Check sheet for the modelled part. Datum: model origin and axes. Units: mm. Face numbers are marked on the shaded views. A direction names the side the tool comes from. Give positions to 0.01 mm unless a question says otherwise; leave off trailing zeros. Order: outer loops, then holes, each group sorted by start corner. A loop starts at its lowest first (then second) coordinate and runs counter-clockwise, first axis right, second up. Notation, with made-up numbers: (3.25, 39) - (14.25, 39) arc R33 ccw to (14.25, 69) - close; hole circle Ø6 at (86, 34.5). An arc over 180 degrees is marked (long way). Answer in a Markdown table with one row per item.
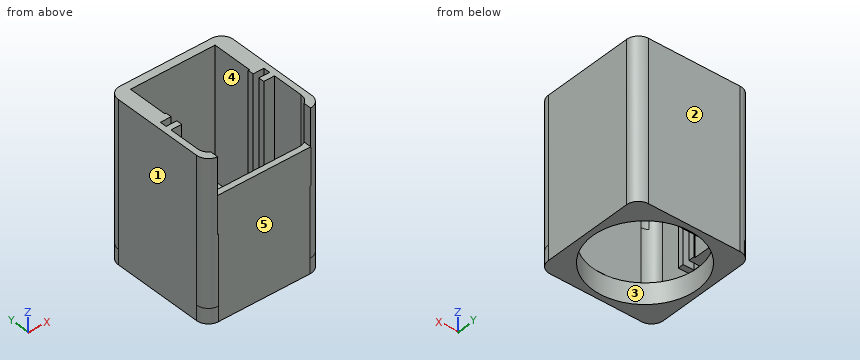
from build123d import *

# Parameters (mm, degrees)
SKETCH1_W            = 100
SKETCH1_H            = 100
BOSS_EXTRUDE1_DEPTH  = 250
SKETCH2_W            = 90
SKETCH2_H            = 90
CUT_EXTRUDE1_DEPTH   = 288.228132327
FILLET1_R            = 10.16
SKETCH3_W            = 9.3412
SKETCH3_H            = 5
BOSS_EXTRUDE2_DEPTH  = 250
SKETCH4_W            = 100
SKETCH4_H            = 125
CUT_EXTRUDE2_DEPTH   = 288.228132327
SKETCH6_W            = 90
SKETCH6_H            = 5.08
BOSS_EXTRUDE3_DEPTH  = 95
SKETCH7_R            = 45.3
CUT_EXTRUDE4_DEPTH   = 5.08
SKETCH10_R           = 48.300000047
BOSS_EXTRUDE4_DEPTH  = 30
SKETCH11_R           = 45.3
CUT_EXTRUDE5_DEPTH   = 30
SKETCH13_W           = 63.5
SKETCH13_H           = 63.5
CUT_EXTRUDE7_DEPTH   = 5
FILLET4_R            = 1.27
FILLET5_R            = 10.16
BOSS_EXTRUDE6_DEPTH  = 30
SKETCH16_R           = 45.3
CUT_EXTRUDE8_DEPTH   = 189.745860882
CUT_EXTRUDE10_DEPTH  = 210.821352584
SKETCH19_W           = 81
SKETCH19_H           = 64.77
CUT_EXTRUDE11_DEPTH  = 25.4
SKETCH20_W           = 81
SKETCH20_H           = 32.5
BOSS_EXTRUDE7_DEPTH  = 5
BOSS_EXTRUDE8_START  = 32.5
BOSS_EXTRUDE8_DEPTH  = 32.5
BOSS_EXTRUDE10_DEPTH = 119.92
SKETCH25_W           = 73.5
SKETCH25_H           = 16.413635584
BOSS_EXTRUDE11_DEPTH = 6.35
SKETCH26_W           = 17
SKETCH26_H           = 125.184112418
CUT_EXTRUDE12_DEPTH  = 288.228132327


with BuildPart() as part:
    # Sketch1 → Boss-Extrude1 (new body)
    with BuildSketch(Plane.XY):
        with Locations((50, 50)):
            Rectangle(SKETCH1_W, SKETCH1_H)
    extrude(amount=BOSS_EXTRUDE1_DEPTH)

    # Sketch2 → Cut-Extrude1 (cut, through all)
    with BuildSketch(Plane(origin=(0, 0, 0), x_dir=(-1, 0, 0), z_dir=(0, 0, -1))):
        with Locations((-50, 50)):
            Rectangle(SKETCH2_W, SKETCH2_H)
    extrude(amount=-CUT_EXTRUDE1_DEPTH, mode=Mode.SUBTRACT)

    # Fillet1
    fillet1_edges = [part.edges().sort_by_distance(p)[0] for p in [
        (0, 100, 125),
        (0, 0, 125),
        (100, 0, 125),
        (100, 100, 125),
    ]]
    fillet(fillet1_edges, radius=FILLET1_R)

    # Sketch3 → Boss-Extrude2 (add, through all)
    with BuildSketch(Plane(origin=(0, 0, 0), x_dir=(-1, 0, 0), z_dir=(0, 0, -1))):
        with Locations((-90.3294, 55.4)):
            Rectangle(SKETCH3_W, SKETCH3_H)
        with Locations((-90.3294, 44.6)):
            Rectangle(SKETCH3_W, SKETCH3_H)
        with Locations((-9.6706, 44.6)):
            Rectangle(SKETCH3_W, SKETCH3_H)
        with Locations((-9.6706, 55.4)):
            Rectangle(SKETCH3_W, SKETCH3_H)
    extrude(amount=-BOSS_EXTRUDE2_DEPTH)

    # Sketch4 → Cut-Extrude2 (cut, through all)
    with BuildSketch(Plane(origin=(0, 100, 0), x_dir=(1, 0, 0), z_dir=(0, 1, 0))):
        with Locations((50, -62.5)):
            Rectangle(SKETCH4_W, SKETCH4_H)
    extrude(amount=-CUT_EXTRUDE2_DEPTH, mode=Mode.SUBTRACT)

    # Sketch6 → Boss-Extrude3 (add)
    with BuildSketch(Plane(origin=(0, 5, 0), x_dir=(1, 0, 0), z_dir=(0, 1, 0))):
        with Locations((50, -127.54)):
            Rectangle(SKETCH6_W, SKETCH6_H)
    extrude(amount=BOSS_EXTRUDE3_DEPTH)

    # Sketch7 → Cut-Extrude4 (cut)
    with BuildSketch(Plane(origin=(0, 0, 125), x_dir=(-1, 0, 0), z_dir=(0, 0, -1))):
        with Locations((-50, 50)):
            Circle(SKETCH7_R)
    extrude(amount=-CUT_EXTRUDE4_DEPTH, mode=Mode.SUBTRACT)

    # Sketch10 → Boss-Extrude4 (add)
    with BuildSketch(Plane(origin=(0, 0, 125), x_dir=(-1, 0, 0), z_dir=(0, 0, -1))):
        with Locations(Location((-50, 50, 0), (0, 0, 180))):
            Circle(SKETCH10_R)
    extrude(amount=BOSS_EXTRUDE4_DEPTH)

    # Sketch11 → Cut-Extrude5 (cut)
    with BuildSketch(Plane(origin=(0, 0, 95), x_dir=(-1, 0, 0), z_dir=(0, 0, -1))):
        with Locations((-50, 50)):
            Circle(SKETCH11_R)
    extrude(amount=-CUT_EXTRUDE5_DEPTH, mode=Mode.SUBTRACT)

    # Sketch13 → Cut-Extrude7 (cut)
    with BuildSketch(Plane.XZ):
        with Locations((50, 218.25)):
            Rectangle(SKETCH13_W, SKETCH13_H)
    extrude(amount=-CUT_EXTRUDE7_DEPTH, mode=Mode.SUBTRACT)

    # Fillet4
    fillet4_edges = [part.edges().sort_by_distance(p)[0] for p in [
        (81.75, 0, 218.25),
        (18.25, 0, 218.25),
        (50, 0, 186.5),
    ]]
    fillet(fillet4_edges, radius=FILLET4_R)

    # Fillet5
    fillet5_edges = [part.edges().sort_by_distance(p)[0] for p in [
        (95, 95, 190.04),
        (5, 95, 190.04),
        (5, 5, 190.04),
        (95, 5, 190.04),
    ]]
    fillet(fillet5_edges, radius=FILLET5_R)

    # Sketch14 → Boss-Extrude6 (add)
    with BuildSketch(Plane(origin=(0, 0, 125), x_dir=(-1, 0, 0), z_dir=(0, 0, -1))):
        with BuildLine():
            Line((-5, 100), (-95, 100))
            Line((-95, 100), (-95, 98.592142595))
            ThreePointArc((-95, 98.592142595), (-98.661881885, 94.879841267), (-100, 89.84))
            Line((-100, 89.84), (-100, 10.16))
            ThreePointArc((-100, 10.16), (-97.024204897, 2.975795103), (-89.84, 0))
            Line((-89.84, 0), (-10.16, 0))
            ThreePointArc((-10.16, 0), (-2.975795103, 2.975795103), (0, 10.16))
            Line((0, 10.16), (0, 89.84))
            ThreePointArc((0, 89.84), (-1.338118115, 94.879841267), (-5, 98.592142595))
            Line((-5, 98.592142595), (-5, 100))
        make_face()
    extrude(amount=BOSS_EXTRUDE6_DEPTH)

    # Sketch16 → Cut-Extrude8 (cut, through all)
    with BuildSketch(Plane.XY.offset(125)):
        with Locations(Location((50, 50, 0), (0, 0, 169.956667322))):
            Circle(SKETCH16_R)
    extrude(amount=-CUT_EXTRUDE8_DEPTH, mode=Mode.SUBTRACT)

    # Sketch18 → Cut-Extrude10 (cut, through all)
    with BuildSketch(Plane(origin=(0, 0, 95), x_dir=(-1, 0, 0), z_dir=(0, 0, -1))):
        with BuildLine():
            Line((-100, 89.84), (-100, 107.62))
            Line((-100, 107.62), (0, 107.62))
            Line((0, 107.62), (0, 89.84))
            ThreePointArc((0, 89.84), (-2.975795103, 97.024204897), (-10.16, 100))
            Line((-10.16, 100), (-89.84, 100))
            ThreePointArc((-89.84, 100), (-97.024204897, 97.024204897), (-100, 89.84))
        make_face()
    extrude(amount=-CUT_EXTRUDE10_DEPTH, mode=Mode.SUBTRACT)

    # Sketch19 → Cut-Extrude11 (cut)
    with BuildSketch(Plane.XZ):
        with Locations((50, 217.615)):
            Rectangle(SKETCH19_W, SKETCH19_H)
    extrude(amount=-CUT_EXTRUDE11_DEPTH, mode=Mode.SUBTRACT)

    # Sketch20 → Boss-Extrude7 (add)
    with BuildSketch(Plane.XZ):
        with Locations((50, 201.48)):
            Rectangle(SKETCH20_W, SKETCH20_H)
    extrude(amount=-BOSS_EXTRUDE7_DEPTH)

    # Sketch21 → Boss-Extrude8 (add)
    with BuildSketch(Plane.XY.offset(185.23).offset(BOSS_EXTRUDE8_START)):
        with BuildLine():
            Line((9.5, 5), (15.16, 5))
            ThreePointArc((15.16, 5), (12.201837845, 5.440181243), (9.5, 6.722583334))
            Line((9.5, 6.722583334), (9.5, 5))
        make_face()
        with BuildLine():
            ThreePointArc((90.5, 6.722583334), (87.798162155, 5.440181243), (84.84, 5))
            Line((84.84, 5), (90.5, 5))
            Line((90.5, 5), (90.5, 6.722583334))
        make_face()
    extrude(amount=-BOSS_EXTRUDE8_DEPTH)

    # Sketch24 → Boss-Extrude10 (add)
    with BuildSketch(Plane.XY.offset(130.08)):
        Polygon((95, 57.9), (86.75, 57.9), (86.75, 92.9), (13.25, 92.9), (13.25, 57.9), (5, 57.9), (5, 95), (95, 95), align=None)
    extrude(amount=BOSS_EXTRUDE10_DEPTH)

    # Sketch25 → Boss-Extrude11 (add)
    with BuildSketch(Plane.XY.offset(130.08)):
        with Locations((50, 84.693182208)):
            Rectangle(SKETCH25_W, SKETCH25_H)
    extrude(amount=BOSS_EXTRUDE11_DEPTH)

    # Sketch26 → Cut-Extrude12 (cut, through all)
    with BuildSketch(Plane(origin=(100, 0, 0), x_dir=(0, 0, -1), z_dir=(1, 0, 0))):
        with Locations((-103.5, 50.164427468)):
            Rectangle(SKETCH26_W, SKETCH26_H)
    extrude(amount=-CUT_EXTRUDE12_DEPTH, mode=Mode.SUBTRACT)


solid = part.part
(1) Thickness scan on L1, parallel to Y at x = 78, z = 152; L2, parallel to X at y = 83.5, z = 163; L3, parallel to X at y = 50, z = 122.25. Record the ranges inside material, lowest first.
Geometry says:
| item | result |
|---|---|
| L1 | 0 to 5, 92.9 to 100 |
| L2 | 0 to 13.25, 86.75 to 100 |
| L3 | 0 to 4.7, 95.3 to 100 |
(2) Mould release check, pull along Y, two halves, no side actions. Record for the marked faces 1, 2 and 3: pulls with the +Y half, pulls with the -Y half, needs draft (parallel to the pull), parting line crosses it, or undercut.
Geometry says:
| item | result |
|---|---|
| face 1 | needs draft |
| face 2 | pulls with the +Y half |
| face 3 | undercut |
(3) Cross-section at B-B, the plane y = 50. Record the cut outline in (x, z), then the cut area to 3 significant figures.
Geometry says:
| item | result |
|---|---|
| outline | (0, 112) - (4.7, 112) - (4.7, 130.08) - (5, 130.08) - (5, 250) - (0, 250) - close; (95, 130.08) - (95.3, 130.08) - (95.3, 112) - (100, 112) - (100, 250) - (95, 250) - close |
| area | 1,370 mm² |
(4) Cross-section at A-A, the plane x = 50. Record the cut outline in (y, z), then the cut area to 3 significant figures.
Geometry says:
| item | result |
|---|---|
| outline | (0, 112) - (4.7, 112) - (4.7, 130.08) - (5, 130.08) - (5, 217.73) - (0, 217.73) - close; (76.49, 130.08) - (95.3, 130.08) - (95.3, 112) - (100, 112) - (100, 250) - (92.9, 250) - (92.9, 136.43) - (76.49, 136.43) - close |
| area | 1,560 mm² |
(5) Access from +Z, -Z, +X, -X, +Y, -Y to the whole of each face (thin tool, end or side, straight path). Record for the marked faces 4 and 5.
Geometry says:
| item | result |
|---|---|
| face 4 | +Z |
| face 5 | +Z, -Z, +X, -X, -Y |
(6) Gauge pin test, flat ends, axial feed: P1, Ø1.5, axis at x = 67, y = 77.5, coming from the +Z side; P2, Ø5.5, axis at x = 67, y = 3.5, coming from the +Z side; P3, Ø3.5, axis at y = 4.5, z = 241.5, coming from the +X side. Record the tip position at first contact, or that the pin passes through.
Geometry says:
| item | result |
|---|---|
| P1 | z = 136.43 |
| P2 | z = 217.73 |
| P3 | x = 99.22 |
